Read the model definition and answer for the solid it produces. Units are mm, in the model's axes. A direction names the side the tool comes from. Round coordinates to 2 decimals unless told otherwise and drop trailing zeros. Write each loop counter-clockwise with the first axis right and the second up, starting at its lowest first coordinate (ties: lowest second). Pieces come first, ordered by that corner, then holes. Notation, with made-up numbers: (-1.75, -22.5) -> (25.25, -22.5) arc R23 ccw to (25.25, -5.5) -> close; hole circle Ø11 at (34.5, 8). An arc over 180 degrees is marked (long way). Return JSON: item names as keys, results as strings. Group by question number.
(1) For faces 1 (the flat face through (75, 7, 49)), 2 (the flat face through (-1, 7, -125)), 3 (the flat face through (-76, 11, -29)), determine the directions among +Z, -Z, +X, -X, +Y, -Y from which every point of the face is accessible in a straight line to the end or side of a thin tool.
(2) A cutting plane is placed at C-C on z = 58.5. Give the vertices of the cut face in (x, y).
(3) A cutting plane is placed at A-A on z = -137.5. Give the vertices of the cut face in (x, y), then the cut area to 3 significant figures.
(4) Given pin 1 (5 mm diameter, centred on y = 6, z = -133.5, fed in from -X); pin 2 (1.5 mm diameter, centred on x = -49, y = 46.5, fed in from -Z); pin 3 (1.2 mm diameter, centred on x = 75, y = 9.5, fed in from -Z), each flat-ended and moving along its own axis, determine where each tip first touches the part or whether it passes through.
(5) Straight lines are drawn through the part: line 1 (Z direction, x = 0, y = 7); line 2 (X direction, y = 6, z = -84); line 3 (Y direction, x = 53, z = 125). For each, find the intervals that lie inside material, in ascending order.
(6) The mould has two halves that part along Z. Classify faces 4 (the flat face through (1, 35, 140)), 5 (the flat face through (-76, 7, 49)), 6 (the flat face through (68, 62, 130)), 7 (the flat face through (78, 9, 34)): released by +Z, released by -Z, zero draft, split by the parting line, or undercut.
(7) A cutting plane is placed at B-B on x = 0. Give the vertices of the cut face in (y, z), then the cut area to 3 significant figures.
(8) A cutting plane is placed at D-D on x = 19. Give the vertices of the cut face in (y, z).
```python
from build123d import *

# Parameters (mm, degrees)
BOSS_EXTRUDE1_DEPTH = 3
BOSS_EXTRUDE2_DEPTH = 8
BOSS_EXTRUDE3_DEPTH = 69
SKETCH4_R           = 4
CUT_EXTRUDE1_DEPTH  = 10
SKETCH5_W           = 5
SKETCH5_H           = 30
CUT_EXTRUDE2_DEPTH  = 4
SKETCH6_W           = 15
SKETCH6_H           = 15
BOSS_EXTRUDE4_DEPTH = 10
SKETCH7_R           = 4
CUT_EXTRUDE3_DEPTH  = 10
FILLET1_R           = 2
SKETCH8_R           = 1.5
CUT_EXTRUDE4_DEPTH  = 286


with BuildPart() as part:
    # Sketch1 → Boss-Extrude1 (new body)
    with BuildSketch(Plane(origin=(0, 0, 0), x_dir=(1, 0, 0), z_dir=(0, 1, 0))):
        Polygon((-78, -130), (-78, -140), (78, -140), (78, -130), (78, 130), (-78, 130), align=None)
    extrude(amount=BOSS_EXTRUDE1_DEPTH)

    # Sketch2 → Boss-Extrude2 (add)
    with BuildSketch(Plane(origin=(0, 3, 0), x_dir=(1, 0, 0), z_dir=(0, 1, 0))):
        Polygon((-73, -120.104101991), (-73, 125), (73, 125), (73, -120.104101991), (78, -120.104101991), (78, 130), (-78, 130), (-78, -120.104101991), align=None)
    extrude(amount=BOSS_EXTRUDE2_DEPTH)

    # Sketch3 → Boss-Extrude3 (add)
    with BuildSketch(Plane(origin=(0, 3, 0), x_dir=(1, 0, 0), z_dir=(0, 1, 0))):
        Polygon((73, -120.104101991), (78, -120.104101991), (78, -140), (-78, -140), (-78, -120.104101991), (-73, -120.104101991), align=None)
    extrude(amount=BOSS_EXTRUDE3_DEPTH)

    # Sketch4 → Cut-Extrude1 (cut)
    with BuildSketch(Plane(origin=(0, 72, 0), x_dir=(1, 0, 0), z_dir=(0, 1, 0))):
        with Locations((-68, -130.104101991)):
            Circle(SKETCH4_R)
        with Locations((68, -130.104101991)):
            Circle(SKETCH4_R)
    extrude(amount=-CUT_EXTRUDE1_DEPTH, mode=Mode.SUBTRACT)

    # Sketch5 → Cut-Extrude2 (cut)
    with BuildSketch(Plane(origin=(0, 11, 0), x_dir=(1, 0, 0), z_dir=(0, 1, 0))):
        with Locations((-75.5, 105)):
            Rectangle(SKETCH5_W, SKETCH5_H)
        with Locations((-75.5, -49.5)):
            Rectangle(SKETCH5_W, SKETCH5_H)
        with Locations((75.5, -49.5)):
            Rectangle(SKETCH5_W, SKETCH5_H)
        with Locations((75.5, 105)):
            Rectangle(SKETCH5_W, SKETCH5_H)
    extrude(amount=-CUT_EXTRUDE2_DEPTH, mode=Mode.SUBTRACT)

    # Sketch6 → Boss-Extrude4 (add)
    with BuildSketch(Plane(origin=(0, 11, 0), x_dir=(1, 0, 0), z_dir=(0, 1, 0))):
        with Locations((0, 137.5)):
            Rectangle(SKETCH6_W, SKETCH6_H)
    extrude(amount=-BOSS_EXTRUDE4_DEPTH)

    # Sketch7 → Cut-Extrude3 (cut)
    with BuildSketch(Plane(origin=(0, 11, 0), x_dir=(1, 0, 0), z_dir=(0, 1, 0))):
        with Locations((0, 137.5)):
            Circle(SKETCH7_R)
    extrude(amount=-CUT_EXTRUDE3_DEPTH, mode=Mode.SUBTRACT)

    # Fillet1
    fillet1_edges = [part.edges().sort_by_distance(p)[0] for p in [
        (7.5, 6, -145),
        (-7.5, 6, -145),
    ]]
    fillet(fillet1_edges, radius=FILLET1_R)

    # Sketch8 → Cut-Extrude4 (cut, through all)
    with BuildSketch(Plane.XY.offset(140)):
        with Locations((53.5, 56)):
            Circle(SKETCH8_R)
        with Locations((53.5, 16)):
            Circle(SKETCH8_R)
        with Locations((-53.5, 16)):
            Circle(SKETCH8_R)
        with Locations((-53.5, 56)):
            Circle(SKETCH8_R)
    extrude(amount=-CUT_EXTRUDE4_DEPTH, mode=Mode.SUBTRACT)


solid = part.part
```
Checks:
{
 "1": {"face 1": "+X, -X, +Y", "face 2": "+Y", "face 3": "-Z, +X, -X, +Y"},
 "2": {"outline": "(-78, 0) -> (78, 0) -> (78, 7) -> (73, 7) -> (73, 3) -> (-73, 3) -> (-73, 7) -> (-78, 7) -> close"},
 "3": {"outline": "(-7.5, 1) -> (-4, 1) -> (-4, 11) -> (-7.5, 11) -> close; (4, 1) -> (7.5, 1) -> (7.5, 11) -> (4, 11) -> close", "area": "70.0 mm^2"},
 "4": {"pin 1": "stops at x = -7.5", "pin 2": "stops at z = 120.1", "pin 3": "stops at z = -130"},
 "5": {"line 1": "z = -145 to -141.5, -133.5 to -125, 120.1 to 140", "line 2": "x = -78 to -73, 73 to 78", "line 3": "y = 0 to 14.59, 17.41 to 54.59, 57.41 to 72"},
 "6": {"face 4": "released by +Z", "face 5": "undercut", "face 6": "undercut", "face 7": "zero draft"},
 "7": {"outline": "(0, -130) -> (1, -130) -> (1, -133.5) -> (11, -133.5) -> (11, -125) -> (3, -125) -> (3, 120.1) -> (72, 120.1) -> (72, 140) -> (0, 140) -> close; (1, -145) -> (11, -145) -> (11, -141.5) -> (1, -141.5) -> close", "area": "2,290 mm^2"},
 "8": {"outline": "(0, -130) -> (11, -130) -> (11, -125) -> (3, -125) -> (3, 120.1) -> (72, 120.1) -> (72, 140) -> (0, 140) -> close"}
}
